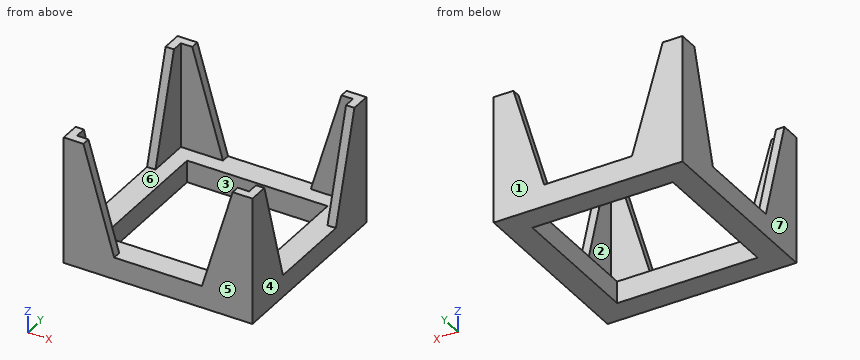
```python
from build123d import *

# Parameters (mm, degrees)
SKETCH_W        = 43
SKETCH_H        = 43
PAD_DEPTH       = 29
SKETCH001_W     = 39.2
SKETCH001_H     = 39.2
POCKET_DEPTH    = 24
SKETCH002_W     = 32
SKETCH002_H     = 32
POCKET001_DEPTH = 5.001
POCKET002_DEPTH = 43.001
POCKET003_DEPTH = 43.001


with BuildPart() as part:
    # Sketch → Pad (new body)
    with BuildSketch(Plane.XY):
        Rectangle(SKETCH_W, SKETCH_H)
    extrude(amount=PAD_DEPTH)

    # Sketch001 → Pocket (cut)
    with BuildSketch(Plane.XY.offset(29)):
        Rectangle(SKETCH001_W, SKETCH001_H)
    extrude(amount=-POCKET_DEPTH, mode=Mode.SUBTRACT)

    # Sketch002 → Pocket001 (cut, through all)
    with BuildSketch(Plane.XY.offset(5)):
        Rectangle(SKETCH002_W, SKETCH002_H)
    extrude(amount=-POCKET001_DEPTH, mode=Mode.SUBTRACT)

    # Sketch003 → Pocket002 (cut, through all)
    with BuildSketch(Plane.XZ.offset(21.5)):
        Polygon((-17, 29), (-10, 5), (10, 5), (17, 29), align=None)
    extrude(amount=-POCKET002_DEPTH, mode=Mode.SUBTRACT)

    # Sketch004 → Pocket003 (cut, through all)
    with BuildSketch(Plane(origin=(-21.5, 0, 0), x_dir=(0, -1, 0), z_dir=(-1, 0, 0))):
        Polygon((-17, 29), (-10, 5), (10, 5), (17, 29), align=None)
    extrude(amount=-POCKET003_DEPTH, mode=Mode.SUBTRACT)


solid = part.part
```
The model under review builds one solid part; all positions refer to its coordinate system, in mm. Face numbers are marked on the shaded views. A direction names the side the tool comes from. Round coordinates to 2 decimals unless told otherwise and drop trailing zeros. Loops run counter-clockwise (first coordinate to the right, second up) from the corner with the lowest first, then second, coordinate; pieces in that order, holes last. Notation, with made-up numbers: (88, 67.25) - (123, 67.25) arc R15 cw to (123, 77.25) - close; hole circle Ø6 at (78, 39.5). An arc over 180 degrees is marked (long way). Use a Markdown table: item, result. Add a question column.
Q1. Insertion check: pin 1 Ø8 at (x, y) = (15, -3) entering from +Z. The pin has a flat end and moves straight along its axis. Give the tip position at first contact, or say it passes through.
Q2. The part is to be moulded in two halves that separate along X. For the marked faces 4, 5, 6 and 7, say which applies: pulls with the +X half, pulls with the -X half, needs draft (parallel to the pull), parting line crosses it, or undercut.
Q3. Add section A-A (x = 2). State the section outline as (y, z) points.
Q4. Add section B-B (z = 23). State the section outline as (x, y) points, plus the area to 3 significant figures.
Q5. Machinability: for the marked faces 1, 2 and 3, which of the approach directions +Z, -Z, +X, -X, +Y, -Y give a long, thin tool a straight path to every point of the face, cutting with its end or side? Answer none if there is none.
Q6. For probe 1 along X at (y, z) = (-8, 2.5); probe 2 along Y at (x, z) = (-15.5, 22.25), list the stretches that pass through material, from the lowest coordinate up.
Q7. Add section D-D (z = 3.5). State the section outline as (x, y) points, plus the area to 3 significant figures.
Worked answers:
| question | item | result |
|---|---|---|
| 1 | pin 1 | z = 5 |
| 2 | face 4 | pulls with the +X half |
| 2 | face 5 | needs draft |
| 2 | face 6 | undercut |
| 2 | face 7 | pulls with the -X half |
| 3 | outline | (-21.5, 0) - (-16, 0) - (-16, 5) - (-21.5, 5) - close; (16, 0) - (21.5, 0) - (21.5, 5) - (16, 5) - close |
| 4 | outline | (-21.5, -21.5) - (-15.25, -21.5) - (-15.25, -19.6) - (-19.6, -19.6) - (-19.6, -15.25) - (-21.5, -15.25) - close; (-21.5, 15.25) - (-19.6, 15.25) - (-19.6, 19.6) - (-15.25, 19.6) - (-15.25, 21.5) - (-21.5, 21.5) - close; (15.25, -21.5) - (21.5, -21.5) - (21.5, -15.25) - (19.6, -15.25) - (19.6, -19.6) - (15.25, -19.6) - close; (15.25, 19.6) - (19.6, 19.6) - (19.6, 15.25) - (21.5, 15.25) - (21.5, 21.5) - (15.25, 21.5) - close |
| 4 | area | 80.6 mm² |
| 5 | face 1 | +Z, -Z, +X, -X, +Y |
| 5 | face 2 | +Z |
| 5 | face 3 | +Z, -Z |
| 6 | probe 1 | -21.5 to -16, 16 to 21.5 |
| 6 | probe 2 | -21.5 to -19.6, 19.6 to 21.5 |
| 7 | outline | (-21.5, -21.5) - (21.5, -21.5) - (21.5, 21.5) - (-21.5, 21.5) - close; hole (-16, -16) - (16, -16) - (16, 16) - (-16, 16) - close |
| 7 | area | 825 mm² |
